Work out the finished part from the listing and answer in its coordinate system (mm). A direction names the side the tool comes from. Coordinates: 2 decimals unless noted, no trailing zeros. Loops run counter-clockwise (first coordinate to the right, second up) from the corner with the lowest first, then second, coordinate; pieces in that order, holes last. Notation, with made-up numbers: (86, 80) -> (144, 80) arc R15 cw to (144, 100) -> close; hole circle Ø4 at (13, 56). An arc over 180 degrees is marked (long way). Use a Markdown table: item, result.
from build123d import *

# Parameters (mm, degrees)
BOSS_EXTRUDE1_DEPTH = 0.5
SKETCH2_R           = 8.575
BOSS_EXTRUDE2_DEPTH = 5
SKETCH3_R           = 1.59
SKETCH3_R_2         = 1.29
CUT_EXTRUDE1_DEPTH  = 4
SKETCH4_R           = 1.7
CUT_EXTRUDE2_DEPTH  = 15.888439307
SKETCH5_R           = 3.1
CUT_EXTRUDE3_DEPTH  = 3.2


with BuildPart() as part:
    # Sketch1 → Boss-Extrude1 (new body)
    with BuildSketch(Plane(origin=(0, 0, 0), x_dir=(1, 0, 0), z_dir=(0, 1, 0))):
        with BuildLine():
            ThreePointArc((8.1, 0), (5.799315036, 6.235382907), (0, 9.482088378))
            ThreePointArc((0, 9.482088378), (-8.1, 0), (0, -9.482088378))
            ThreePointArc((0, -9.482088378), (5.799315036, -6.235382907), (8.1, 0))
        make_face()
    extrude(amount=BOSS_EXTRUDE1_DEPTH)

    # Sketch2 → Boss-Extrude2 (add)
    with BuildSketch(Plane(origin=(0, 0.5, 0), x_dir=(1, 0, 0), z_dir=(0, 1, 0))):
        with Locations(Location((-1.5, 0, 0), (0, 0, 100.787083295))):
            Circle(SKETCH2_R)
    extrude(amount=BOSS_EXTRUDE2_DEPTH)

    # Sketch3 → Cut-Extrude1 (cut)
    with BuildSketch(Plane(origin=(0, 0, 0), x_dir=(1, 0, 0), z_dir=(0, 1, 0))):
        with Locations(Location((0, 5.8, 0), (0, 0, 270))):
            Circle(SKETCH3_R)
        with Locations(Location((0, -5.8, 0), (0, 0, 270))):
            Circle(SKETCH3_R_2)
    extrude(amount=CUT_EXTRUDE1_DEPTH, mode=Mode.SUBTRACT)

    # Sketch4 → Cut-Extrude2 (cut, through all)
    with BuildSketch(Plane(origin=(0, 5.5, 0), x_dir=(1, 0, 0), z_dir=(0, 1, 0))):
        with Locations(Location((0, 0, 0), (0, 0, 270))):
            Circle(SKETCH4_R)
    extrude(amount=-CUT_EXTRUDE2_DEPTH, mode=Mode.SUBTRACT)

    # Sketch5 → Cut-Extrude3 (cut)
    with BuildSketch(Plane(origin=(0, 5.5, 0), x_dir=(1, 0, 0), z_dir=(0, 1, 0))):
        with Locations(Location((0, 0, 0), (0, 0, 270))):
            Circle(SKETCH5_R)
    extrude(amount=-CUT_EXTRUDE3_DEPTH, mode=Mode.SUBTRACT)


solid = part.part
Q1. Given pin 1 Ø1.6 at (x, z) = (0, -6.5) entering from -Y; pin 2 Ø1.5 at (y, z) = (3.5, -7) entering from -X; pin 3 Ø2 at (y, z) = (2.5, -2) entering from +X, each flat-ended and moving along its own axis, determine where each tip first touches the part or whether it passes through.
Solved:
| item | result |
|---|---|
| pin 1 | y = 4 |
| pin 2 | x = -7.37 |
| pin 3 | x = 7.02 |
Q2. Section A-A on z = 5.8 is taken. Determine the outline of the cut face in (x, y), and give its area (3 significant figures).
Solved:
| item | result |
|---|---|
| outline | (-7.82, 0.5) -> (-6.15, 0.5) -> (-6.15, 0) -> (-1.29, 0) -> (-1.29, 4) -> (1.29, 4) -> (1.29, 0) -> (6.15, 0) -> (6.15, 0.5) -> (4.82, 0.5) -> (4.82, 5.5) -> (-7.82, 5.5) -> close |
| area | 59.0 mm² |
Q3. Section B-B on y = 1.5 is taken. Determine the outline of the cut face in (x, z) (3 decimals), and give its area (3 significant figures).
Solved:
| item | result |
|---|---|
| outline | circle Ø17.15 at (-1.5, 0); hole circle Ø3.4 at (0, 0); hole circle Ø3.18 at (0, -5.8); hole circle Ø2.58 at (0, 5.8) |
| area | 209 mm² |
Q4. Consider line 1 (Z direction, x = -0.25, y = 2.9); line 2 (Z direction, x = 0.5, y = 0.55); line 3 (X direction, y = 4.05, z = 0) (3 decimals). Determine where each line is inside the solid, lowest interval first. Write a range as [from, to].
Solved:
| item | result |
|---|---|
| line 1 | [-8.48, -7.37], [-4.23, -3.09], [3.09, 4.53], [7.07, 8.48] |
| line 2 | [-8.34, -7.31], [-4.29, -1.62], [1.62, 4.61], [6.99, 8.34] |
| line 3 | [-10.075, -3.1], [3.1, 7.075] |
Q5. Determine the mould class of faces 1 (the cylindrical face through (0.39, 1.97, 7.03)), 2 (the cylindrical face through (-5.561, 2.965, -7.552)), 3 (the cylindrical face through (-8.1, 0.25, -0.19)) for opening direction X: pulls with the +X half, pulls with the -X half, needs draft (parallel to the pull), parting line crosses it, or undercut.
Solved:
| item | result |
|---|---|
| face 1 | undercut |
| face 2 | parting line crosses it |
| face 3 | pulls with the -X half |
Q6. Section C-C on z = 0.25 is taken. Determine the outline of the cut face in (x, y).
Solved:
| item | result |
|---|---|
| outline | (-10.07, 0.5) -> (-8.1, 0.5) -> (-8.1, 0) -> (-1.68, 0) -> (-1.68, 2.3) -> (-3.09, 2.3) -> (-3.09, 5.5) -> (-10.07, 5.5) -> close; (1.68, 0) -> (8.1, 0) -> (8.1, 0.5) -> (7.07, 0.5) -> (7.07, 5.5) -> (3.09, 5.5) -> (3.09, 2.3) -> (1.68, 2.3) -> close |
Q7. Section D-D on x = -6 is taken. Determine the outline of the cut face in (y, z), and give its area (3 significant figures).
Solved:
| item | result |
|---|---|
| outline | (0, -5.99) -> (0.5, -5.99) -> (0.5, -7.3) -> (5.5, -7.3) -> (5.5, 7.3) -> (0.5, 7.3) -> (0.5, 5.99) -> (0, 5.99) -> close |
| area | 79.0 mm² |
Q8. For faces 4 (the cylindrical face through (0.931, 3.922, 2.957)), 5 (the cylindrical face through (-1.66, 1.17, -0.37)), 6 (the cylindrical face through (-0.61, 1.97, -4.33)), 7 (the flat face through (-2, 0, 0)), 8 (the flat face through (-8.4, 0.5, 0.4)), determine the directions among +Z, -Z, +X, -X, +Y, -Y from which every point of the face is accessible in a straight line to the end or side of a thin tool.
Solved:
| item | result |
|---|---|
| face 4 | +Y |
| face 5 | +Y, -Y |
| face 6 | -Y |
| face 7 | +Z, -Z, +X, -X, -Y |
| face 8 | -X, -Y |
